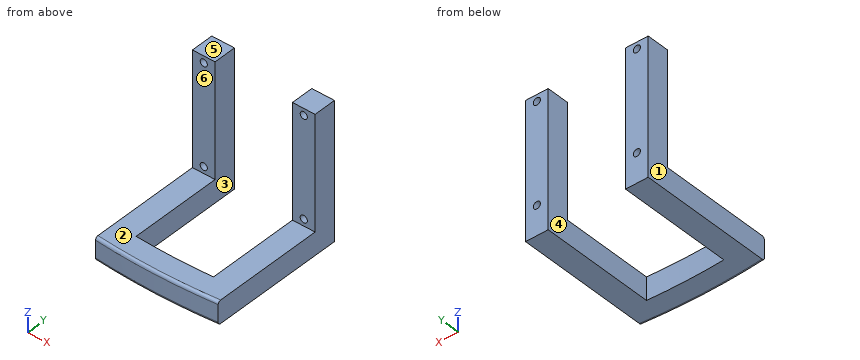
from build123d import *

# Parameters (mm, degrees)
F0_W     = 6.35
F0_H     = 6.341725
F2_DEPTH = 6.35
F1_W     = 6.35
F1_H     = 6.35
F3_DEPTH = 38.1
F5_D     = 2
F6_R     = 0.79375


with BuildPart() as f2:
    # F0 (on Top) → F2 (new body)
    with BuildSketch(Plane.XY):
        with BuildLine():
            Line((-10.825, 5.877161), (-10.825, 0))
            Line((-10.825, 0), (-17.175, 0))
            ThreePointArc((-17.175, 0), (0, -0.802674), (17.175, 0))
            Line((17.175, 0), (10.825, 0))
            Line((10.825, 0), (10.825, 5.877161))
            ThreePointArc((10.825, 5.877161), (0, 5.547326), (-10.825, 5.877161))
        make_face()
        Polygon((-17.175, 0), (-10.825, 0), (-10.825, 5.877161), (-10.825, 31.758275), (-17.175, 31.758275), align=None)
        with Locations((-14, 34.929137)):
            Rectangle(F0_W, F0_H)
        Polygon((10.825, 0), (17.175, 0), (17.175, 31.758275), (10.825, 31.758275), (10.825, 5.877161), align=None)
        with Locations((14, 34.929137)):
            Rectangle(F0_W, F0_H)
    extrude(amount=F2_DEPTH)

    # F1 (on Top) → F3 (join)
    with BuildSketch(Plane.XY):
        with Locations((-14, 34.925)):
            Rectangle(F1_W, F1_H)
        with Locations((14, 34.925)):
            Rectangle(F1_W, F1_H)
    extrude(amount=F3_DEPTH)

    # F5 (through all)
    with Locations(Plane.XZ.offset(-31.75)):
        with Locations((-14, 36.225), (-14, 8.225), (14, 8.225), (14, 36.225)):
            Hole(F5_D / 2)

    # F6
    f6_edges = [f2.edges().sort_by_distance(p)[0] for p in [
        (0, -0.802674, 6.35),
        (0, -0.802674, 0),
    ]]
    fillet(f6_edges, radius=F6_R)


solid = f2.part
Work out the finished part from the listing and answer in its coordinate system (mm). Face numbers are marked on the shaded views. A direction names the side the tool comes from. Give positions to 0.01 mm unless a question says otherwise; leave off trailing zeros. Loops run counter-clockwise (first coordinate to the right, second up) from the corner with the lowest first, then second, coordinate; pieces in that order, holes last. Notation, with made-up numbers: M -22.5,81.25 L 13.5,81.25 A37 cw 13.5,119.25 Z; hole C 76.25,82 d2. An arc over 180 degrees is marked long. Use CSV: the item, a comma, the result in double quotes.
1) Find section D-D on x = 0. Write down the section's boundary in (y, z), plus the area to 3 significant figures.
Answer:
outline,"M -0.8,0.79 A0.79 ccw -0.01,0 L 5.55,0 L 5.55,6.35 L -0.01,6.35 A0.79 ccw -0.8,5.56 Z"
area,"40.1 mm^2"
2) Find section B-B on y = 34.5. Write down the section's boundary in (x, z) (3 decimals).
Answer:
outline,"M -17.175,0 L -10.825,0 L -10.825,38.1 L -17.175,38.1 Z; M 10.825,0 L 17.175,0 L 17.175,38.1 L 10.825,38.1 Z; hole C -14,8.225 d2; hole C -14,36.225 d2; hole C 14,8.225 d2; hole C 14,36.225 d2"
3) Find section C-C on y = 10. Write down the section's boundary in (x, z) (3 decimals).
Answer:
outline,"M -17.175,0 L -10.825,0 L -10.825,6.35 L -17.175,6.35 Z; M 10.825,0 L 17.175,0 L 17.175,6.35 L 10.825,6.35 Z"
4) Determine the mould class of the marked faces 1, 2, 3 and 4 for opening direction X: released by +X, released by -X, zero draft, split by the parting line, or undercut.
Answer:
face 1,"released by -X"
face 2,"zero draft"
face 3,"undercut"
face 4,"undercut"
5) Consider L1, parallel to Z at x = 14, y = 34.5 (3 decimals); L2, parallel to X at y = 36, z = 5 (3 decimals); L3, parallel to Z at x = 13.5, y = 32. Determine where each line is inside the solid, lowest interval first.
Answer:
L1,"0 to 7.225, 9.225 to 35.225, 37.225 to 38.1"
L2,"-17.175 to -10.825, 10.825 to 17.175"
L3,"0 to 7.36, 9.09 to 35.36, 37.09 to 38.1"
6) Which of the six approach directions +Z, -Z, +X, -X, +Y, -Y give full straight-line access (tool end or side, diameter ignored) to the marked faces 5 and 6?
Answer:
face 5,"+Z, +X, -X, +Y, -Y"
face 6,"+Z, +X, -X, -Y"
7) Given P1, Ø16, axis at x = 7, y = 19, coming from the +Z side; P2, Ø3, axis at x = 12.5, z = 16.5, coming from the -Y side, each flat-ended and moving along its own axis, determine where each tip first touches the part or whether it passes through.
Answer:
P1,"z = 6.35"
P2,"y = 31.75"
8) Find section A-A on z = 16. Write down the section's boundary in (x, y) (3 decimals).
Answer:
outline,"M -17.175,31.75 L -10.825,31.75 L -10.825,38.1 L -17.175,38.1 Z; M 10.825,31.75 L 17.175,31.75 L 17.175,38.1 L 10.825,38.1 Z"
